Work out the finished part from the listing and answer in its coordinate system (mm). Face numbers are marked on the shaded views. A direction names the side the tool comes from. Round coordinates to 2 decimals unless told otherwise and drop trailing zeros. Write each loop counter-clockwise with the first axis right and the second up, starting at its lowest first coordinate (ties: lowest second). Pieces come first, ordered by that corner, then holes. Notation, with made-up numbers: (28.5, 35.25) - (50.5, 35.25) arc R28 ccw to (50.5, 73.25) - close; hole circle Ø9 at (69, 3.5). An arc over 180 degrees is marked (long way). Answer as a JSON object with one key per item and string values.
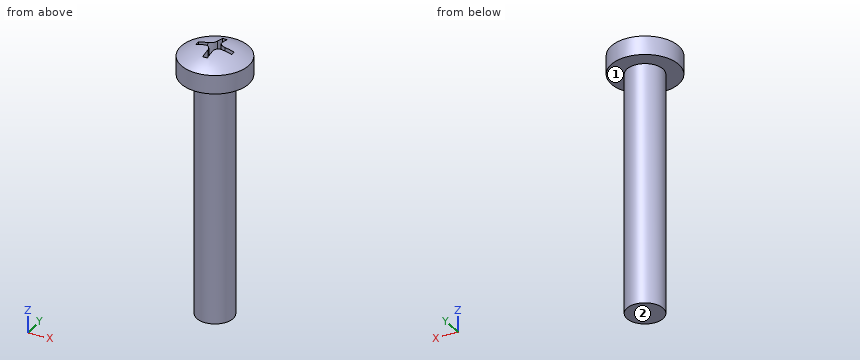
```python
from build123d import *

# Parameters (mm, degrees)
SKETCH1_R          = 1.5
BASE_EXTRUDE_DEPTH = 20
CUT_EXTRUDE1_DEPTH = 1.799999969
CUT_EXTRUDE1_TAPER = 2


with BuildPart() as part:
    # Sketch1 → Base-Extrude (new body)
    with BuildSketch(Plane.XY):
        Circle(SKETCH1_R)
    extrude(amount=BASE_EXTRUDE_DEPTH)

    # Sketch6 → Boss-Revolve2 (revolve)
    with BuildSketch(Plane(origin=(0, 0, 0), x_dir=(1, 0, 0), z_dir=(0, 1, 0)), mode=Mode.PRIVATE) as boss_revolve2_sk:
        with BuildLine():
            Line((0, -20), (2.7999999, -20))
            Line((2.7999999, -20), (2.7999999, -21.54246308))
            ThreePointArc((2.7999999, -21.54246308), (1.46418655, -22.180811406), (0, -22.4))
            Line((0, -22.4), (0, -20))
        make_face()
    revolve(boss_revolve2_sk.sketch.rotate(Axis((0, 0, -0.393620135), (0, 0, 1)), 180), axis=Axis((0, 0, -0.393620135), (0, 0, 1)))

    # Sketch7 → Cut-Extrude1 (cut)
    with BuildSketch(Plane(origin=(0, 0, 22.7000001), x_dir=(-1, 0, 0), z_dir=(0, 0, -1))):
        with BuildLine():
            ThreePointArc((0.205000004, 1.48592565), (0, 1.500000013), (-0.205000004, 1.48592565))
            Line((-0.205000004, 1.48592565), (-0.205000004, 0.708178558))
            ThreePointArc((-0.205000004, 0.708178558), (-0.35072876, 0.355344481), (-0.702967546, 0.208182689))
            Line((-0.702967546, 0.208182689), (-1.48592565, 0.205000004))
            ThreePointArc((-1.48592565, 0.205000004), (-1.500000013, 0), (-1.48592565, -0.205000004))
            Line((-1.48592565, -0.205000004), (-0.702967546, -0.208182689))
            ThreePointArc((-0.702967546, -0.208182689), (-0.35072876, -0.355344481), (-0.205000004, -0.708178558))
            Line((-0.205000004, -0.708178558), (-0.205000004, -1.48592565))
            ThreePointArc((-0.205000004, -1.48592565), (0, -1.500000013), (0.205000004, -1.48592565))
            Line((0.205000004, -1.48592565), (0.205000004, -0.708178558))
            ThreePointArc((0.205000004, -0.708178558), (0.35072876, -0.355344481), (0.702967546, -0.208182689))
            Line((0.702967546, -0.208182689), (1.48592565, -0.205000004))
            ThreePointArc((1.48592565, -0.205000004), (1.500000013, 0), (1.48592565, 0.205000004))
            Line((1.48592565, 0.205000004), (0.702967546, 0.208182689))
            ThreePointArc((0.702967546, 0.208182689), (0.35072876, 0.355344481), (0.205000004, 0.708178558))
            Line((0.205000004, 0.708178558), (0.205000004, 1.48592565))
        make_face()
    extrude(amount=CUT_EXTRUDE1_DEPTH, taper=CUT_EXTRUDE1_TAPER, mode=Mode.SUBTRACT)


solid = part.part
```
Item 1: A cutting plane is placed at A-A (z = 11.75). Write down the section's boundary in (x, y), and give its area (3 significant figures).
Results found:
{"outline": "circle Ø3 at (0, 0)", "area": "7.07 mm²"}
Item 2: Each of these flat-tipped pins is pushed along its axis until it touches: P1, Ø3, axis at x = -1, z = 3, coming from the -Y side; P2, Ø2, axis at x = -1.5, y = 2, coming from the +Z side; P3, Ø2, axis at y = -2, z = 11.5, coming from the +X side. Where does it stop, or does it pass through?
Results found:
{"P1": "y = -1.5", "P2": "z = 22.17", "P3": "x = 1.12"}
Item 3: Consider line 1 along X through (y, z) = (-0.05, 2.25); line 2 along Y through (x, z) = (0.45, 17.75); line 3 along Y through (x, z) = (-0.2, 16.5). Determine where each line is inside the solid, lowest interval first.
Results found:
{"line 1": "-1.5 to 1.5", "line 2": "-1.43 to 1.43", "line 3": "-1.49 to 1.49"}
Item 4: For the marked faces 1 and 2, determine the directions among +Z, -Z, +X, -X, +Y, -Y from which every point of the face is accessible in a straight line to the end or side of a thin tool.
Results found:
{"face 1": "-Z", "face 2": "-Z, +X, -X, +Y, -Y"}
Item 5: A cutting plane is placed at B-B (x = 1.9). Write down the section's boundary in (y, z), and give its area (3 significant figures).
Results found:
{"outline": "(-2.06, 20) - (2.06, 20) - (2.06, 21.54) arc R4.62 ccw to (-2.06, 21.54) - close", "area": "7.68 mm²"}
